Geometry check sheet. Reference: the model listing, model coordinates, mm. Face numbers are marked on the shaded views. Coordinates: 2 decimals unless noted, no trailing zeros. Write each loop counter-clockwise with the first axis right and the second up, starting at its lowest first coordinate (ties: lowest second). Pieces come first, ordered by that corner, then holes. Notation, with made-up numbers: M 69,58 L 88,58 A18 cw 88,83 Z; hole C -20,-16 d2. An arc over 180 degrees is marked long. Write item = value, one per line. Start each with the question number.
```python
from build123d import *

# Parameters (mm, degrees)
F2_R     = 4.7625
F3_DEPTH = 9.525
F4_R     = 1.5875
F5_DEPTH = 17.145


with BuildPart() as f1:
    # F0 (on Front) → F1 (revolve)
    with BuildSketch(Plane.XZ):
        with BuildLine():
            Line((0, 63.5), (0, 0))
            Line((0, 0), (23.876184, 4.954478))
            ThreePointArc((23.876184, 4.954478), (27.511198, 7.163922), (28.935999, 11.172028))
            Line((28.935999, 11.172028), (28.935999, 57.15))
            ThreePointArc((28.935999, 57.15), (27.076127, 61.640128), (22.585999, 63.5))
            Line((22.585999, 63.5), (0, 63.5))
        make_face()
    revolve(axis=Axis((0, 0, 31.75), (0, 0, -1)))

    # F2 (on face) → F3 (cut)
    with BuildSketch(Plane.XY.offset(63.5)):
        Circle(F2_R)
    extrude(amount=-F3_DEPTH, mode=Mode.SUBTRACT)

    # F4 (on Top) → F5 (cut)
    with BuildSketch(Plane.XY):
        Circle(F4_R)
    extrude(amount=F5_DEPTH, mode=Mode.SUBTRACT)


solid = f1.part
```
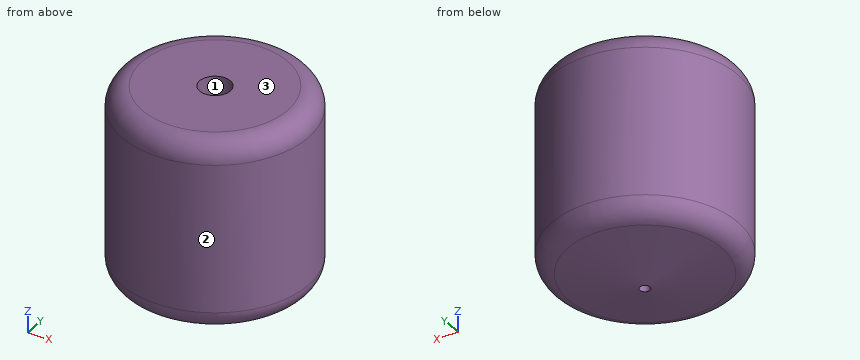
Q1. Scan lines: L1, parallel to Y at x = 0, z = 56.5; L2, parallel to X at y = 0, z = 11; L3, parallel to X at y = -4, z = 60. Record each from-to range of solid material in increasing order.
Q2. Cross-section at C-C on z = 56. Enter the section's corners in (x, y) (1 decimal), and give its area (3 significant figures).
Q3. Draft check along Y on the marked faces 1, 2 and 3. Enter one of: pulls with the +Y half, pulls with the -Y half, needs draft (parallel to the pull), parting line crosses it, or undercut.
Q4. Gauge pin test, flat ends, axial feed: pin 1 (1 mm diameter, centred on y = -10.5, z = 57, fed in from -X); pin 2 (4 mm diameter, centred on x = 6, z = 10, fed in from -Y); pin 3 (12 mm diameter, centred on y = 16.5, z = 16.5, fed in from +X). Record the tip position at first contact, or that the pin passes through.
Q5. Cross-section at D-D on z = 18.5. Enter the section's corners in (x, y), and give its area (3 significant figures).
Values found:
q1.L1 = -28.94 to -4.76, 4.76 to 28.94
q1.L2 = -28.93 to -1.59, 1.59 to 28.93
q1.L3 = -27.98 to -2.58, 2.58 to 27.98
q2.outline = C 0,0 d57.9; hole C 0,0 d9.5
q2.area = 2,560 mm²
q3.face_1 = undercut
q3.face_2 = parting line crosses it
q3.face_3 = needs draft
q4.pin_1 = -27.15
q4.pin_2 = -28.62
q4.pin_3 = 26.96
q5.outline = C 0,0 d57.87
q5.area = 2,630 mm²
